The figure shows three views and two pictorial views of one solid part (mm, origin at its lowest corner). Answer the questions. Round coordinates to 2 decimals unless told otherwise and drop trailing zeros. Loops run counter-clockwise (first coordinate to the right, second up) from the corner with the lowest first, then second, coordinate; pieces in that order, holes last. Notation, with made-up numbers: (-22, 28.5) -> (-18, 28.5) arc R21 cw to (-18, 48.5) -> close; hole circle Ø10 at (54.25, 50). An arc over 180 degrees is marked (long way). Write item = value, one per line. Start each with the question number.
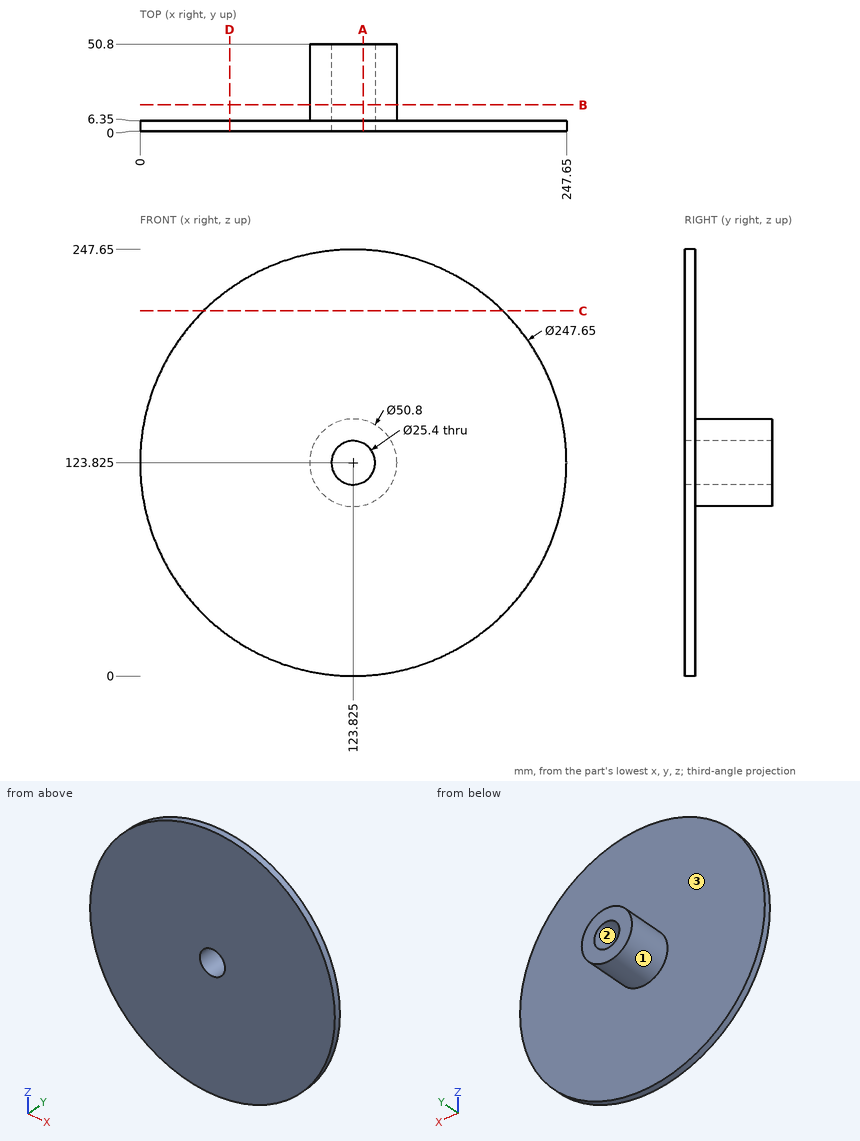
Item 1: Section B-B (y = 15.5) is taken. Determine the outline of the cut face in (x, z) (3 decimals).
Item 2: Section A-A (x = 129.5) is taken. Determine the outline of the cut face in (y, z).
Item 3: Section D-D (x = 52) is taken. Determine the outline of the cut face in (y, z).
Item 4: Flat-ended cylindrical pins translate along their axes: pin 1 (2 mm diameter, centred on x = 151.5, y = 14, fed in from +Z); pin 2 (12 mm diameter, centred on y = 44.5, z = 113.5, fed in from -X); pin 3 (4 mm diameter, centred on x = 112, y = 14.5, fed in from +Z). Find the tip coordinate at first contact, or state that the pin passes through.
Item 5: Find the intervals of material crossed by line 1 along Y through (x, z) = (43.5, 46); line 2 along X through (y, z) = (2.5, 203.5); line 3 along X through (y, z) = (3, 102), in increasing order. Write a range as [from, to].
Item 6: Section C-C (z = 212) is taken. Determine the outline of the cut face in (x, y), then the cut area to 3 significant figures.
Item 7: The mould has two halves that part along Z. Classify the marked faces 1, 2 and 3: pulls with the +Z half, pulls with the -Z half, needs draft (parallel to the pull), parting line crosses it, or undercut.
Worked answers:
q1.outline = circle Ø50.8 at (123.825, 123.825); hole circle Ø25.4 at (123.825, 123.825)
q2.outline = (0, 0.13) -> (6.35, 0.13) -> (6.35, 99.07) -> (50.8, 99.07) -> (50.8, 112.46) -> (0, 112.46) -> close; (0, 135.19) -> (50.8, 135.19) -> (50.8, 148.58) -> (6.35, 148.58) -> (6.35, 247.52) -> (0, 247.52) -> close
q3.outline = (0, 22.96) -> (6.35, 22.96) -> (6.35, 224.69) -> (0, 224.69) -> close
q4.pin_1 = through
q4.pin_2 = 98.8
q4.pin_3 = 147.25
q5.line_1 = [0, 6.35]
q5.line_2 = [29.04, 218.61]
q5.line_3 = [1.94, 245.71]
q6.outline = (36.89, 0) -> (210.76, 0) -> (210.76, 6.35) -> (36.89, 6.35) -> close
q6.area = 1,100 mm2
q7.face_1 = parting line crosses it
q7.face_2 = undercut
q7.face_3 = needs draft
